```python
from build123d import *

# Parameters (mm, degrees)
F1_DEPTH  = 1066.8
F2_W      = 812.8
F2_H      = 660.4
F3_DEPTH  = 19.05
F4_W      = 812.8
F4_H      = 660.4
F4_W_2    = 774.7
F4_H_2    = 622.3
F5_DEPTH  = 152.4
F6_W      = 76.2
F6_H      = 76.2
F7_DEPTH  = 660.401
F8_W      = 76.2
F8_H      = 76.2
F9_DEPTH  = 812.801
F10_W     = 571.5
F10_H     = 19.05
F11_DEPTH = 438.15
F12_W     = 571.5
F12_H     = 19.05
F13_DEPTH = 495.3


with BuildPart() as f1:
    # F0 (on Front) → F1 (new body, symmetric)
    with BuildSketch(Plane.XZ):
        Polygon((304.8, -228.6), (304.8, 228.6), (285.75, 228.6), (285.75, 209.55), (285.75, -209.55), (-285.75, -209.55), (-285.75, 209.55), (-285.75, 228.6), (-304.8, 228.6), (-304.8, -228.6), align=None)
    extrude(amount=F1_DEPTH, both=True)

    # F2 (on face) → F3 (join)
    with BuildSketch(Plane.XZ.offset(1066.8)):
        Rectangle(F2_W, F2_H)
    extrude(amount=F3_DEPTH)

    # F4 (on face) → F5 (join)
    with BuildSketch(Plane.XZ.offset(1085.85)):
        Rectangle(F4_W, F4_H)
        Rectangle(F4_W_2, F4_H_2, mode=Mode.SUBTRACT)
    extrude(amount=F5_DEPTH)

    # F6 (on face) → F7 (cut, through all)
    with BuildSketch(Plane(origin=(0, 0, -330.2), x_dir=(1, 0, 0), z_dir=(0, 0, -1))):
        with Locations((-304.8, 1200.15)):
            Rectangle(F6_W, F6_H)
        with Locations((-152.4, 1200.15)):
            Rectangle(F6_W, F6_H)
        with Locations((0, 1200.15)):
            Rectangle(F6_W, F6_H)
        with Locations((152.4, 1200.15)):
            Rectangle(F6_W, F6_H)
        with Locations((304.8, 1200.15)):
            Rectangle(F6_W, F6_H)
    extrude(amount=-F7_DEPTH, mode=Mode.SUBTRACT)

    # F8 (on face) → F9 (cut, through all)
    with BuildSketch(Plane(origin=(-406.4, 0, 0), x_dir=(0, -1, 0), z_dir=(-1, 0, 0))):
        with Locations((1200.15, 228.6)):
            Rectangle(F8_W, F8_H)
        with Locations((1200.15, 76.2)):
            Rectangle(F8_W, F8_H)
        with Locations((1200.15, -76.2)):
            Rectangle(F8_W, F8_H)
        with Locations((1200.15, -228.6)):
            Rectangle(F8_W, F8_H)
    extrude(amount=-F9_DEPTH, mode=Mode.SUBTRACT)

    # F10 (on face) → F11 (join, through all)
    with BuildSketch(Plane.XY.offset(-209.55)):
        with Locations((0, 1057.275)):
            Rectangle(F10_W, F10_H)
    extrude(amount=F11_DEPTH)

    # F12 (on face) → F13 (join)
    with BuildSketch(Plane(origin=(0, -1066.8, 0), x_dir=(-1, 0, 0), z_dir=(0, 1, 0))):
        with Locations((0, 219.075)):
            Rectangle(F12_W, F12_H)
    extrude(amount=F13_DEPTH)


solid = f1.part
```
Geometry check sheet. Reference: the model listing, model coordinates, mm. A direction names the side the tool comes from. Round coordinates to 2 decimals unless told otherwise and drop trailing zeros. Write each loop counter-clockwise with the first axis right and the second up, starting at its lowest first coordinate (ties: lowest second). Pieces come first, ordered by that corner, then holes. Notation, with made-up numbers: (7.5, -18) - (49.5, -18) arc R24 cw to (49.5, 3) - close; hole circle Ø6 at (1.5, 69.5). An arc over 180 degrees is marked (long way). Write each question's results on one line, items separated by ' | '.
(1) Set-up check for faces 5 (the face through (-285.75, -24, 6)), 6 (the face through (387.35, -1144, -4)), 7 (the face through (-4, -15, -228.6)): record each of +Z, -Z, +X, -X, +Y, -Y from which the full face is reachable in a straight line by a thin tool's end or side.
Computed:
face 5: none | face 6: -Y | face 7: -Z, +X, -X, +Y
(2) Draft check along Y on faces 1 (the face through (-5, -1085.85, 4)), 2 (the face through (-5, -1144, -311.15)), 3 (the face through (-4, -1066.8, 3)), 4 (the face through (285.75, -24, 13)). Enter one of: pulls with the +Y half, pulls with the -Y half, needs draft (parallel to the pull), parting line crosses it, or undercut.
Computed:
face 1: pulls with the -Y half | face 2: needs draft | face 3: undercut | face 4: undercut
(3) Sectioned sample at B-B, the plane z = -61.5. Enter the section's corners in (x, y).
Computed:
outline: (-406.4, -1162.05) - (-387.35, -1162.05) - (-387.35, -1085.85) - (387.35, -1085.85) - (387.35, -1162.05) - (406.4, -1162.05) - (406.4, -1066.8) - (304.8, -1066.8) - (304.8, 1066.8) - (-304.8, 1066.8) - (-304.8, -1066.8) - (-406.4, -1066.8) - close; hole (-285.75, -1066.8) - (285.75, -1066.8) - (285.75, 1047.75) - (-285.75, 1047.75) - close
(4) Sectioned sample at A-A, the plane y = -791.5. Enter the section's corners in (x, z).
Computed:
outline: (-304.8, -228.6) - (304.8, -228.6) - (304.8, 228.6) - (-304.8, 228.6) - close; hole (-285.75, -209.55) - (285.75, -209.55) - (285.75, 209.55) - (-285.75, 209.55) - close
(5) Sectioned sample at C-C, the plane x = -215.5. Enter the section's corners in (y, z), plus the area to 3 significant figures.
Computed:
outline: (-1238.25, -330.2) - (-1066.8, -330.2) - (-1066.8, -228.6) - (1066.8, -228.6) - (1066.8, 228.6) - (1047.75, 228.6) - (1047.75, -209.55) - (-1066.8, -209.55) - (-1066.8, 209.55) - (-571.5, 209.55) - (-571.5, 228.6) - (-1066.8, 228.6) - (-1066.8, 330.2) - (-1238.25, 330.2) - (-1238.25, 311.15) - (-1085.85, 311.15) - (-1085.85, -311.15) - (-1238.25, -311.15) - close | area: 76,800 mm^2
(6) Depth check by flat-ended pin: pin 1 Ø2 at (y, z) = (-315, -150) entering from -X; pin 2 Ø4 at (x, z) = (85.5, -236.5) entering from -Y; pin 3 Ø1 at (y, z) = (237.5, -200) entering from +X. Enter the tip coordinate at first touch or a pass-through.
Computed:
pin 1: stops at x = -304.8 | pin 2: stops at y = -1085.85 | pin 3: stops at x = 304.8
(7) Sectioned sample at D-D, the plane y = -80. Enter the section's corners in (x, z), plus the area to 3 significant figures.
Computed:
outline: (-304.8, -228.6) - (304.8, -228.6) - (304.8, 228.6) - (285.75, 228.6) - (285.75, -209.55) - (-285.75, -209.55) - (-285.75, 228.6) - (-304.8, 228.6) - close | area: 28,300 mm^2
(8) Thickness scan on probe 1 along Y at (x, z) = (196.5, -77); probe 2 along X at (y, z) = (181, 188); probe 3 along X at (y, z) = (-1090, 28). Record the ranges inside material, lowest first. Write a range as from..to.
Computed:
probe 1: y = -1085.85..-1066.8, 1047.75..1066.8 | probe 2: x = -304.8..-285.75, 285.75..304.8 | probe 3: x = -406.4..-387.35, 387.35..406.4
